Build history of the part. All positions in model axes, mm. A direction names the side the tool comes from. Round coordinates to 2 decimals unless told otherwise and drop trailing zeros. Write each loop counter-clockwise with the first axis right and the second up, starting at its lowest first coordinate (ties: lowest second). Pieces come first, ordered by that corner, then holes.
Autodesk Inventor part; units mm, degrees
ref_plane "YZ Plane" through (0, 0, 0) normal (1, 0, 0) x (0, 1, 0)
ref_plane "XZ Plane" through (0, 0, 0) normal (0, 1, 0) x (-1, 0, 0)
ref_plane "XY Plane" through (0, 0, 0) normal (0, 0, 1) x (1, 0, 0)
sketch "Sketch1" plane through (0, 0, 0) normal (0, 1, 0) x (-1, 0, 0)
  circle A0 centre (0, 0) radius 144.3
  circle A1 centre (0, 0) radius 153.3
  dimension "d1" = 9
  dimension "d5" = 306.6
extrude "Extrusion1" add sketch "Sketch1" along normal blind 4
sketch "Sketch2" plane through (0, 4, 0) normal (0, 1, 0) x (1, 0, 0)
  line L0 (0, 0) -> (143.7298, 38.5123) construction
  line L1 (146.1384, 40.9209) -> (147.0201, 37.6306)
  line L2 (147.0201, 37.6306) -> (144.6114, 35.222)
  line L3 (144.6114, 35.222) -> (141.3211, 36.1036)
  line L4 (141.3211, 36.1036) -> (140.4395, 39.3939)
  line L5 (140.4395, 39.3939) -> (142.8481, 41.8026)
  line L6 (142.8481, 41.8026) -> (146.1384, 40.9209)
  line L7 (0, 0) -> (153.3, 0) construction
  circle A0 centre (0, 0) radius 153.3
  line L8 (102.8088, 107.6262) -> (106.0991, 108.5078)
  line L9 (101.9272, 104.3359) -> (102.8088, 107.6262)
  line L10 (104.3359, 101.9272) -> (101.9272, 104.3359)
  line L11 (107.6262, 102.8088) -> (104.3359, 101.9272)
  line L12 (108.5078, 106.0991) -> (107.6262, 102.8088)
  line L13 (106.0991, 108.5078) -> (108.5078, 106.0991)
  line L14 (35.222, 144.6114) -> (37.6306, 147.0201)
  line L15 (36.1036, 141.3211) -> (35.222, 144.6114)
  line L16 (39.3939, 140.4395) -> (36.1036, 141.3211)
  line L17 (41.8026, 142.8481) -> (39.3939, 140.4395)
  line L18 (40.9209, 146.1384) -> (41.8026, 142.8481)
  line L19 (37.6306, 147.0201) -> (40.9209, 146.1384)
  line L20 (-41.8026, 142.8481) -> (-40.9209, 146.1384)
  line L21 (-39.3939, 140.4395) -> (-41.8026, 142.8481)
  line L22 (-36.1036, 141.3211) -> (-39.3939, 140.4395)
  line L23 (-35.222, 144.6114) -> (-36.1036, 141.3211)
  line L24 (-37.6306, 147.0201) -> (-35.222, 144.6114)
  line L25 (-40.9209, 146.1384) -> (-37.6306, 147.0201)
  line L26 (-107.6262, 102.8088) -> (-108.5078, 106.0991)
  line L27 (-104.3359, 101.9272) -> (-107.6262, 102.8088)
  line L28 (-101.9272, 104.3359) -> (-104.3359, 101.9272)
  line L29 (-102.8088, 107.6262) -> (-101.9272, 104.3359)
  line L30 (-106.0991, 108.5078) -> (-102.8088, 107.6262)
  line L31 (-108.5078, 106.0991) -> (-106.0991, 108.5078)
  line L32 (-144.6114, 35.222) -> (-147.0201, 37.6306)
  line L33 (-141.3211, 36.1036) -> (-144.6114, 35.222)
  line L34 (-140.4395, 39.3939) -> (-141.3211, 36.1036)
  line L35 (-142.8481, 41.8026) -> (-140.4395, 39.3939)
  line L36 (-146.1384, 40.9209) -> (-142.8481, 41.8026)
  line L37 (-147.0201, 37.6306) -> (-146.1384, 40.9209)
  line L38 (-142.8481, -41.8026) -> (-146.1384, -40.9209)
  line L39 (-140.4395, -39.3939) -> (-142.8481, -41.8026)
  line L40 (-141.3211, -36.1036) -> (-140.4395, -39.3939)
  line L41 (-144.6114, -35.222) -> (-141.3211, -36.1036)
  line L42 (-147.0201, -37.6306) -> (-144.6114, -35.222)
  line L43 (-146.1384, -40.9209) -> (-147.0201, -37.6306)
  line L44 (-102.8088, -107.6262) -> (-106.0991, -108.5078)
  line L45 (-101.9272, -104.3359) -> (-102.8088, -107.6262)
  line L46 (-104.3359, -101.9272) -> (-101.9272, -104.3359)
  line L47 (-107.6262, -102.8088) -> (-104.3359, -101.9272)
  line L48 (-108.5078, -106.0991) -> (-107.6262, -102.8088)
  line L49 (-106.0991, -108.5078) -> (-108.5078, -106.0991)
  line L50 (-35.222, -144.6114) -> (-37.6306, -147.0201)
  line L51 (-36.1036, -141.3211) -> (-35.222, -144.6114)
  line L52 (-39.3939, -140.4395) -> (-36.1036, -141.3211)
  line L53 (-41.8026, -142.8481) -> (-39.3939, -140.4395)
  line L54 (-40.9209, -146.1384) -> (-41.8026, -142.8481)
  line L55 (-37.6306, -147.0201) -> (-40.9209, -146.1384)
  line L56 (41.8026, -142.8481) -> (40.9209, -146.1384)
  line L57 (39.3939, -140.4395) -> (41.8026, -142.8481)
  line L58 (36.1036, -141.3211) -> (39.3939, -140.4395)
  line L59 (35.222, -144.6114) -> (36.1036, -141.3211)
  line L60 (37.6306, -147.0201) -> (35.222, -144.6114)
  line L61 (40.9209, -146.1384) -> (37.6306, -147.0201)
  line L62 (107.6262, -102.8088) -> (108.5078, -106.0991)
  line L63 (104.3359, -101.9272) -> (107.6262, -102.8088)
  line L64 (101.9272, -104.3359) -> (104.3359, -101.9272)
  line L65 (102.8088, -107.6262) -> (101.9272, -104.3359)
  line L66 (106.0991, -108.5078) -> (102.8088, -107.6262)
  line L67 (108.5078, -106.0991) -> (106.0991, -108.5078)
  line L68 (144.6114, -35.222) -> (147.0201, -37.6306)
  line L69 (141.3211, -36.1036) -> (144.6114, -35.222)
  line L70 (140.4395, -39.3939) -> (141.3211, -36.1036)
  line L71 (142.8481, -41.8026) -> (140.4395, -39.3939)
  line L72 (146.1384, -40.9209) -> (142.8481, -41.8026)
  line L73 (147.0201, -37.6306) -> (146.1384, -40.9209)
  dimension "d6" = 148.8
  dimension "d7" = 5.9
  dimension "d8" = 15
  dimension "d11" = 360
extrude "Extrusion2" cut sketch "Sketch2" against normal blind 2 contours L1 L2 L3 L4 L5 L6 | L8 L13 L12 L11 L10 L9 | L14 L19 L18 L17 L16 L15 | L20 L25 L24 L23 L22 L21 | L26 L31 L30 L29 L28 L27 | L32 L37 L36 L35 L34 L33 | L38 L43 L42 L41 L40 L39 | L44 L49 L48 L47 L46 L45 | L50 L55 L54 L53 L52 L51 | L56 L61 L60 L59 L58 L57 | L62 L67 L66 L65 L64 L63 | L68 L73 L72 L71 L70 L69
sketch "Sketch3" plane through (0, 2, 0) normal (0, 1, 0) x (1, 0, 0)
  circle A0 centre (143.7298, 38.5123) radius 1.7
  line L0 (144.6114, 35.222) -> (141.3211, 36.1036)
  line L1 (142.8481, 41.8026) -> (146.1384, 40.9209)
  line L2 (144.6114, 35.222) -> (142.8481, 41.8026) construction
  circle A1 centre (105.2175, 105.2175) radius 1.7
  circle A2 centre (38.5123, 143.7298) radius 1.7
  circle A3 centre (-38.5123, 143.7298) radius 1.7
  circle A4 centre (-105.2175, 105.2175) radius 1.7
  circle A5 centre (-143.7298, 38.5123) radius 1.7
  circle A6 centre (-143.7298, -38.5123) radius 1.7
  circle A7 centre (-105.2175, -105.2175) radius 1.7
  circle A8 centre (-38.5123, -143.7298) radius 1.7
  circle A9 centre (38.5123, -143.7298) radius 1.7
  circle A10 centre (105.2175, -105.2175) radius 1.7
  circle A11 centre (143.7298, -38.5123) radius 1.7
  point P0 (0, 0)
  dimension "d15" = 3.4
  dimension "d18" = 360
extrude "Extrusion3" cut sketch "Sketch3" against normal through all
properties part number "ArmLoopOuterRing"
1) Slice it at A-A (x = 0). Write the cut outline in (y, z).
Results:
outline: (0, -153.3) - (4, -153.3) - (4, -144.3) - (0, -144.3) - close; (0, 144.3) - (4, 144.3) - (4, 153.3) - (0, 153.3) - close
2) Pin check, flat tips, straight feed: pin 1 Ø4 at (x, z) = (-143.73, 38.51) entering from +Y; pin 2 Ø2 at (y, z) = (2, -12) entering from +X. Stop position of each tip, or through.
Results:
pin 1: stops at y = 2
pin 2: stops at x = 152.9
3) Which spindle directions (+Z, -Z, +X, -X, +Y, -Y) get a long thin tool onto all of the face, cutting with end or side? Do faces 1 (the flat face through (-40, 2, 142)), 2 (the flat face through (-113, 4, -90)). Say none if no direction does.
Results:
face 1: +Y
face 2: +Z, -Z, +X, -X, +Y
4) Slice it at B-B (z = 0). Write the cut outline in (x, y), plus the area to 3 significant figures.
Results:
outline: (-153.3, 0) - (-144.3, 0) - (-144.3, 4) - (-153.3, 4) - close; (144.3, 0) - (153.3, 0) - (153.3, 4) - (144.3, 4) - close
area: 72.0 mm2
5) Wall check: L1, parallel to X at y = 2.85, z = -3.5; L2, parallel to Z at x = -28, y = 2.55; L3, parallel to X at y = 2.35, z = 56.5. Give the ranges that are in metal, low to high.
Results:
L1: x = -153.26 to -144.26, 144.26 to 153.26
L2: z = -150.72 to -141.56, 141.56 to 150.72
L3: x = -142.51 to -132.78, 132.78 to 142.51
6) Mould opens along Z. For faces 3 (the flat face through (-113, 0, -90)), 4 (the cylindrical face through (33.232, 1.972, 149.655)), 5 (the flat face through (-145, 2, 40)) say: released by +Z, released by -Z, zero draft, split by the parting line, or undercut.
Results:
face 3: zero draft
face 4: split by the parting line
face 5: undercut
7) Slice it at C-C (y = 3.1). Count the separate pieces of the cut face and the enclosed holes in it, plus the area to 3 significant figures.
Results:
separate pieces: 1
enclosed holes: 13
area: 8,050 mm2
